Design review of the part built by this model. Coordinates are the model's own, in mm. Face numbers are marked on the shaded views. Round coordinates to 2 decimals unless told otherwise and drop trailing zeros. Order: outer loops, then holes, each group sorted by start corner. A loop starts at its lowest first (then second) coordinate and runs counter-clockwise, first axis right, second up.
from build123d import *

# Parameters (mm, degrees)
CHAMFER1_SIZE  = 1
CHAMFER1_SIZE2 = 0.577350269


with BuildPart() as part:
    # Sketch1 → Revolve1 (revolve)
    with BuildSketch(Plane.XY, mode=Mode.PRIVATE) as revolve1_sk:
        Polygon((16, 2), (9, 2), (8.75, 2), (8.75, 17), (6.75, 17), (6.75, 2), (0, 2), (0, 0), (16, 0), align=None)
    revolve(revolve1_sk.sketch.rotate(Axis((0, 21.623043933, 0), (0, -1, 0)), 90), axis=Axis((0, 21.623043933, 0), (0, -1, 0)))

    # Chamfer1
    chamfer1_edges = [part.edges().sort_by_distance(p)[0] for p in [
        (0, 17, -8.75),
    ]]
    chamfer1_side = [part.faces().sort_by_distance(p)[0] for p in [
        (0, 9.5, -8.75),
    ]]
    chamfer(chamfer1_edges, length=CHAMFER1_SIZE, length2=CHAMFER1_SIZE2, reference=chamfer1_side[0])


solid = part.part
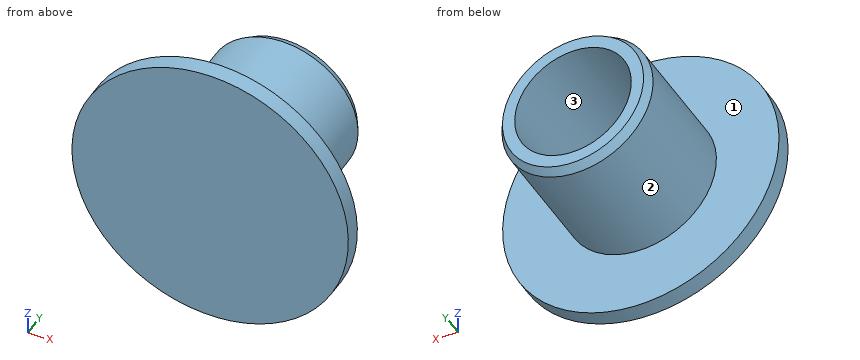
1) Take a section at B-B on y = 4.5. Give the boundary of the cut face in (x, z), plus the area to 3 significant figures.
Results:
outline: circle Ø17.5 at (0, 0); hole circle Ø13.5 at (0, 0)
area: 97.4 mm2
2) The part is to be moulded in two halves that separate along Z. For the marked faces 1, 2 and 3, say which applies: released by +Z, released by -Z, zero draft, split by the parting line, or undercut.
Results:
face 1: zero draft
face 2: split by the parting line
face 3: undercut
3) To check wall thickness, follow line 1 along X through (y, z) = (12, 0); line 2 along Y through (x, z) = (-5, 13); line 3 along X through (y, z) = (10.5, -2.5). State the ranges of each line that lie inside material, in increasing order.
Results:
line 1: x = -8.75 to -6.75, 6.75 to 8.75
line 2: y = 0 to 2
line 3: x = -8.39 to -6.27, 6.27 to 8.39
4) Clearance check with flat-ended pins moving along their axes: P1, Ø1, axis at y = 5.5, z = 7, coming from the -X side; P2, Ø4, axis at y = 7.5, z = -1.5, coming from the -X side; P3, Ø8, axis at x = 8, z = 10, coming from the +Y side. State where each tip first meets the part, or that it passes through.
Results:
P1: stops at x = -5.86
P2: stops at x = -8.75
P3: stops at y = 2
5) Take a section at A-A on x = 0. Give the boundary of the cut face in (y, z), plus the area to 3 significant figures.
Results:
outline: (0, -16) - (2, -16) - (2, -8.75) - (16, -8.75) - (17, -8.17) - (17, -6.75) - (2, -6.75) - (2, 6.75) - (17, 6.75) - (17, 8.17) - (16, 8.75) - (2, 8.75) - (2, 16) - (0, 16) - close
area: 123 mm2
6) Take a section at D-D on x = 13. Give the boundary of the cut face in (y, z).
Results:
outline: (0, -9.33) - (2, -9.33) - (2, 9.33) - (0, 9.33) - close
7) Take a section at C-C on z = 0. Give the boundary of the cut face in (x, y), plus the area to 3 significant figures.
Results:
outline: (-16, 0) - (16, 0) - (16, 2) - (8.75, 2) - (8.75, 16) - (8.17, 17) - (6.75, 17) - (6.75, 2) - (-6.75, 2) - (-6.75, 17) - (-8.17, 17) - (-8.75, 16) - (-8.75, 2) - (-16, 2) - close
area: 123 mm2
